For this review, take the finished solid that the model builds, in its own axes (mm). Face numbers are marked on the shaded views. A direction names the side the tool comes from. Give positions to 0.01 mm unless a question says otherwise; leave off trailing zeros. Order: outer loops, then holes, each group sorted by start corner. A loop starts at its lowest first (then second) coordinate and runs counter-clockwise, first axis right, second up. Notation, with made-up numbers: (-18.75, 14.25) - (8.25, 14.25) arc R20 ccw to (8.25, 23.25) - close; hole circle Ø7 at (67, 46). An arc over 180 degrees is marked (long way). Answer as a JSON object with one key per item and string values. Group by question number.
Autodesk Inventor part; units mm, degrees
ref_plane "YZ Plane" through (0, 0, 0) normal (1, 0, 0) x (0, 1, 0)
ref_plane "XZ Plane" through (0, 0, 0) normal (0, 1, 0) x (-1, 0, 0)
ref_plane "XY Plane" through (0, 0, 0) normal (0, 0, 1) x (1, 0, 0)
sketch "스케치1" plane through (0, 0, 0) normal (0, 0, 1) x (1, 0, 0)
  line L0 (-2, 22.5) -> (2, 22.5)
  line L1 (2, 22.5) -> (2, -22.5)
  line L2 (2, -22.5) -> (-2, -22.5)
  line L3 (-2, -22.5) -> (-2, 22.5)
  point P0 (0, 0)
  dimension "d0" = 4
  dimension "d1" = 45
  dimension "d2" = 2
  dimension "d3" = 22.5
extrude "돌출1" add sketch "스케치1" along normal blind 34
sketch "스케치2" plane through (0, 0, 34) normal (0, 0, 1) x (1, 0, 0)
  circle A0 centre (0, 15) radius 1
  circle A1 centre (0, 7.5) radius 1
  circle A2 centre (0, -7.5) radius 1
  circle A3 centre (0, -15) radius 1
  line L0 (2, 22.5) -> (-2, 22.5)
  line L1 (-2, 22.5) -> (-2, -22.5)
  line L2 (-2, -22.5) -> (2, -22.5)
  line L3 (2, -22.5) -> (2, 22.5)
  circle A4 centre (0, 0) radius 1
  point P0 (0, 0)
  dimension "d6" = 2
  dimension "d7" = 2
  dimension "d8" = 2
  dimension "d9" = 2
  dimension "d11" = 2
  dimension "d12" = 2
  dimension "d13" = 2
  dimension "d14" = 2
  dimension "d17" = 7.5
  dimension "d18" = 7.5
  dimension "d20" = 7.5
  dimension "d21" = 2
  dimension "d22" = 2
  dimension "d23" = 7.5
  dimension "d26" = 7.5
  dimension "d27" = 7.5
extrude "돌출3" cut sketch "스케치2" against normal blind 8 contours A0 | A1 | A2 | A3 | A4
sketch "스케치3" plane through (0, 0, 0) normal (0, 0, -1) x (-1, 0, 0)
  circle A0 centre (0, -15) radius 1
  circle A1 centre (0, 7.5) radius 1
  circle A2 centre (0, 15) radius 1
  circle A3 centre (0, -7.5) radius 1
  circle A4 centre (0, 0) radius 1
  line L0 (-2, 22.5) -> (2, 22.5)
  line L1 (2, 22.5) -> (2, -22.5)
  line L2 (2, -22.5) -> (-2, -22.5)
  line L3 (-2, -22.5) -> (-2, 22.5)
  point P0 (0, 0)
extrude "돌출4" cut sketch "스케치3" against normal blind 8 contours A0 | A1 | A2 | A3 | A4
sketch "스케치4" plane through (-2, -22.5, 0) normal (-1, 0, 0) x (0, 0, 1)
  line L0 (0, 0) -> (0, 45)
  line L1 (0, 0) -> (34, 0)
  line L2 (34, 45) -> (34, 0)
  line L3 (0, 45) -> (34, 45)
  line L4 (8, 36.5) -> (8, 38.5)
  line L5 (26, 38.5) -> (26, 36.5)
  line L6 (12.5, 33) -> (21.5, 33)
  line L7 (21.5, 33) -> (21.5, 12)
  line L8 (21.5, 12) -> (12.5, 12)
  line L9 (12.5, 12) -> (12.5, 33)
  point P0 (0, 22.5)
  dimension "d32" = 12
  dimension "d33" = 21
  dimension "d34" = 9
  dimension "d35" = 12.5
  dimension "d36" = 34
  dimension "d37" = 12.5
  dimension "d40" = 45
  dimension "d41" = 12
extrude "돌출5" cut sketch "스케치4" against normal up to surface (4 mm away) contours L6 L7 L8 L9
fillet "모깎기1" radius 2.5 4 edges at (0, 10.5, 12.5) (0, 10.5, 21.5) (0, -10.5, 12.5) (0, -10.5, 21.5)
equation "\"d35\" = -0.5 * d34 + 0.5 * d36"
properties part number "Box_Side" material "LCP 플라스틱"
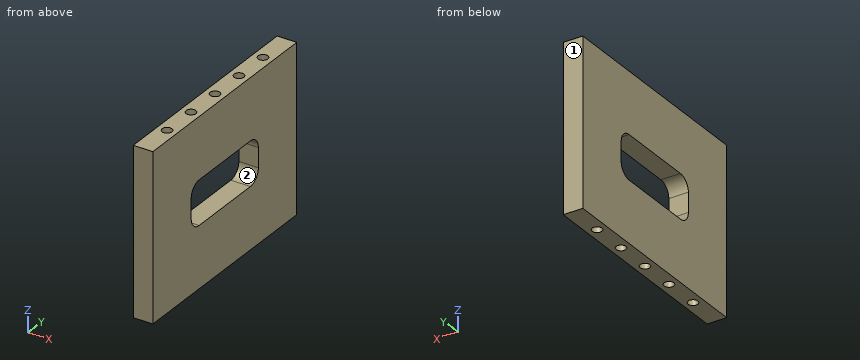
1) Consider section B-B (z = 16). Give the boundary of the cut face in (x, y), plus the area to 3 significant figures.
2) For pin 1 (0.6 mm diameter, centred on x = 0, y = -8, fed in from +Z); pin 2 (0.6 mm diameter, centred on x = 0, y = 0, fed in from -Z), all flat-tipped, find the tip position at first contact; note any pin that passes through.
3) Consider section C-C (z = 26.5). Give the boundary of the cut face in (x, y).
4) Consider section A-A (y = 7.5). Give the boundary of the cut face in (x, z).
5) For line 1 (Y direction, x = 0, z = 30.25); line 2 (Y direction, x = 0.6, z = 19); line 3 (Y direction, x = 0.85, z = 4), list the stretches that pass through material, from the lowest coordinate up.
6) For the marked faces 1 and 2, list the 3-axis set-ups (+Z, -Z, +X, -X, +Y, -Y) from which the entire face can be reached by the end or side of a thin tool; tool diameter is ignored.
7) Consider section D-D (y = -15). Give the boundary of the cut face in (x, z), plus the area to 3 significant figures.
Result set:
{
 "1": {"outline": "(-2, -22.5) - (2, -22.5) - (2, -10.5) - (-2, -10.5) - close; (-2, 10.5) - (2, 10.5) - (2, 22.5) - (-2, 22.5) - close", "area": "96.0 mm2"},
 "2": {"pin 1": "stops at z = 26", "pin 2": "stops at z = 8"},
 "3": {"outline": "(-2, -22.5) - (2, -22.5) - (2, 22.5) - (-2, 22.5) - close; hole circle Ø2 at (0, -15); hole circle Ø2 at (0, -7.5); hole circle Ø2 at (0, 0); hole circle Ø2 at (0, 7.5); hole circle Ø2 at (0, 15)"},
 "4": {"outline": "(-2, 0) - (-1, 0) - (-1, 8) - (1, 8) - (1, 0) - (2, 0) - (2, 12.5) - (-2, 12.5) - close; (-2, 21.5) - (2, 21.5) - (2, 34) - (1, 34) - (1, 26) - (-1, 26) - (-1, 34) - (-2, 34) - close"},
 "5": {"line 1": "y = -22.5 to -16, -14 to -8.5, -6.5 to -1, 1 to 6.5, 8.5 to 14, 16 to 22.5", "line 2": "y = -22.5 to -10.5, 10.5 to 22.5", "line 3": "y = -22.5 to -15.53, -14.47 to -8.03, -6.97 to -0.53, 0.53 to 6.97, 8.03 to 14.47, 15.53 to 22.5"},
 "6": {"face 1": "+Z, -Z, +X, -X, +Y", "face 2": "+X, -X"},
 "7": {"outline": "(-2, 0) - (-1, 0) - (-1, 8) - (1, 8) - (1, 0) - (2, 0) - (2, 34) - (1, 34) - (1, 26) - (-1, 26) - (-1, 34) - (-2, 34) - close", "area": "104 mm2"}
}
